from build123d import *

# Parameters (mm, degrees)
F0_R     = 1.25
F1_DEPTH = 1.25
F2_SIZE  = 0.2


with BuildPart() as f1:
    # F0 (on Right) → F1 (new body, symmetric)
    with BuildSketch(Plane.YZ):
        with BuildLine():
            Line((2.5, -11.5), (2.5, 11.5))
            ThreePointArc((2.5, 11.5), (0, 14), (-2.5, 11.5))
            Line((-2.5, 11.5), (-2.5, -11.5))
            ThreePointArc((-2.5, -11.5), (0, -14), (2.5, -11.5))
        make_face()
        with Locations((0, -11.5)):
            Circle(F0_R, mode=Mode.SUBTRACT)
        with Locations((0, 11.5)):
            Circle(F0_R, mode=Mode.SUBTRACT)
    extrude(amount=F1_DEPTH, both=True)

    # F2
    f2_edges = [f1.edges().sort_by_distance(p)[0] for p in [
        (1.25, 2.5, 0),
        (1.25, 0, 14),
        (1.25, -2.5, 0),
        (1.25, 0, -14),
        (-1.25, 0, 14),
        (-1.25, 2.5, 0),
        (-1.25, -2.5, 0),
        (-1.25, 0, -14),
        (-1.25, -1.25, 11.5),
        (-1.25, -1.25, -11.5),
        (1.25, -1.25, 11.5),
        (1.25, -1.25, -11.5),
    ]]
    chamfer(f2_edges, length=F2_SIZE)


solid = f1.part
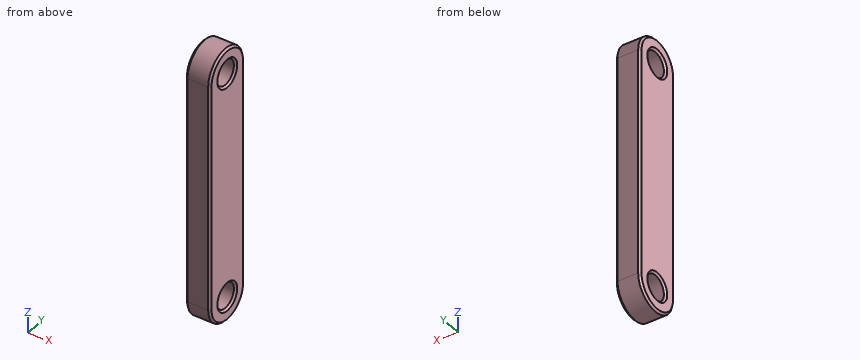
Here's how the part is built. I have some questions about the finished solid (model axes, mm). Coordinates: 2 decimals unless noted, no trailing zeros. Order: outer loops, then holes, each group sorted by start corner. A loop starts at its lowest first (then second) coordinate and runs counter-clockwise, first axis right, second up. Notation, with made-up numbers: M -9.5,69.25 L 29.5,69.25 A28 cw 29.5,106.25 Z; hole C -21.5,-23 d5. An arc over 180 degrees is marked long. Answer as CSV lines item,"result".
Item 1: Imagine slicing it at A-A on y = 0. Write out the boundary of the cut face in (x, z).
Results found:
outline,"M -1.25,-13.8 L -1.05,-14 L 1.05,-14 L 1.25,-13.8 L 1.25,-12.95 L 1.05,-12.75 L -1.05,-12.75 L -1.25,-12.95 Z; M -1.25,-10.05 L -1.05,-10.25 L 1.05,-10.25 L 1.25,-10.05 L 1.25,10.05 L 1.05,10.25 L -1.05,10.25 L -1.25,10.05 Z; M -1.25,12.95 L -1.05,12.75 L 1.05,12.75 L 1.25,12.95 L 1.25,13.8 L 1.05,14 L -1.05,14 L -1.25,13.8 Z"
Item 2: Imagine slicing it at B-B on x = 0.5. Write out the boundary of the cut face in (y, z).
Results found:
outline,"M -2.5,-11.5 A2.5 ccw 2.5,-11.5 L 2.5,11.5 A2.5 ccw -2.5,11.5 Z; hole C 0,-11.5 d2.5; hole C 0,11.5 d2.5"
Item 3: If I drill on line 1 (Z direction, x = -0.05, y = 0); line 2 (Z direction, x = -0.65, y = -0.7); line 3 (Y direction, x = -0.05, z = -10.5), over which ranges is the centre line in solid material (lowest first)?
Results found:
line 1,"-14 to -12.75, -10.25 to 10.25, 12.75 to 14"
line 2,"-13.9 to -12.54, -10.46 to 10.46, 12.54 to 13.9"
line 3,"-2.5 to -0.75, 0.75 to 2.5"
